Autodesk Fusion 360 part; units mm, degrees
sketch "Sketch1" plane through (0, 0, 0) normal (0, 1, 0) x (1, 0, 0)
  circle A0 centre (0, 0) radius 30
  circle A1 centre (0, 0) radius 27
  dimension "d1" = 60
  dimension "d7" = 3
extrude "Extrude1" add sketch "Sketch1" along normal blind 100 makes body 1
extrude "Extrude2" add sketch "Sketch1" along normal blind 4 contours A1 bodies 1
copy_body "Body->Comp1" bodies 1 removing the originals makes body 2 in component "tubeToolHolder03"
component "tubeToolHolder03" placed x (1, 0, 0) y (0, 1, 0) z (0, 0, 1) at (0, 0, 0)
Check sheet for the modelled part. Datum: model origin and axes. Units: mm. Give positions to 0.01 mm unless a question says otherwise; leave off trailing zeros. Loops run counter-clockwise (first coordinate to the right, second up) from the corner with the lowest first, then second, coordinate; pieces in that order, holes last. Notation, with made-up numbers: M 28,-35 L 60,-35 A32 ccw 60,-4 Z; hole C 75.25,-34.5 d3. An arc over 180 degrees is marked long. Return JSON: item names as keys, results as strings. Group by question number.
1. Go/stop test with flat-tipped pins: pin 1 (5 mm diameter, centred on y = 11.5, z = 3.5, fed in from +X); pin 2 (6 mm diameter, centred on x = 2, y = 68.5, fed in from -Z); pin 3 (3 mm diameter, centred on x = 6, y = 51.5, fed in from +Z). Record where each tip stops, or that it passes through.
2. Thickness scan on L1, parallel to Z at x = 1, y = 34.5; L2, parallel to X at y = 60, z = 0; L3, parallel to X at y = 45.5, z = -14.5. Record the ranges inside material, lowest first.
3. Cross-section at B-B on z = 0. Record the boundary of the cut face in (x, y), plus the area to 3 significant figures.
4. Mould release check, pull along Z, two halves, no side actions. Record for faces 1 (the cylindrical face through (-29.97, 49.3, 1.32)), 2 (the cylindrical face through (-5.85, 51.33, -26.36)), 3 (the flat face through (-25, 100, -11)), 4 (the flat face through (0, 4, 0)): released by +Z, released by -Z, zero draft, split by the parting line, or undercut.
5. Cross-section at A-A on x = 0. Record the boundary of the cut face in (y, z), plus the area to 3 significant figures.
6. Cross-section at C-C on y = 6. Record the boundary of the cut face in (x, z).
Return value:
{
 "1": {"pin 1": "x = 29.98", "pin 2": "z = -30", "pin 3": "z = 29.66"},
 "2": {"L1": "-29.98 to -26.98, 26.98 to 29.98", "L2": "-30 to -27, 27 to 30", "L3": "-26.26 to -22.78, 22.78 to 26.26"},
 "3": {"outline": "M -30,0 L 30,0 L 30,100 L 27,100 L 27,4 L -27,4 L -27,100 L -30,100 Z", "area": "816 mm^2"},
 "4": {"face 1": "split by the parting line", "face 2": "undercut", "face 3": "zero draft", "face 4": "undercut"},
 "5": {"outline": "M 0,-30 L 100,-30 L 100,-27 L 4,-27 L 4,27 L 100,27 L 100,30 L 0,30 Z", "area": "816 mm^2"},
 "6": {"outline": "C 0,0 d60; hole C 0,0 d54"}
}
